Input: dimensioned drawing with shaded views. Units: mm. Origin: part minimum x, y, z. A direction names the side the tool comes from. Give positions to 0.01 mm unless a question says otherwise; leave off trailing zeros. Order: outer loops, then holes, each group sorted by start corner. A loop starts at its lowest first (then second) coordinate and runs counter-clockwise, first axis right, second up.
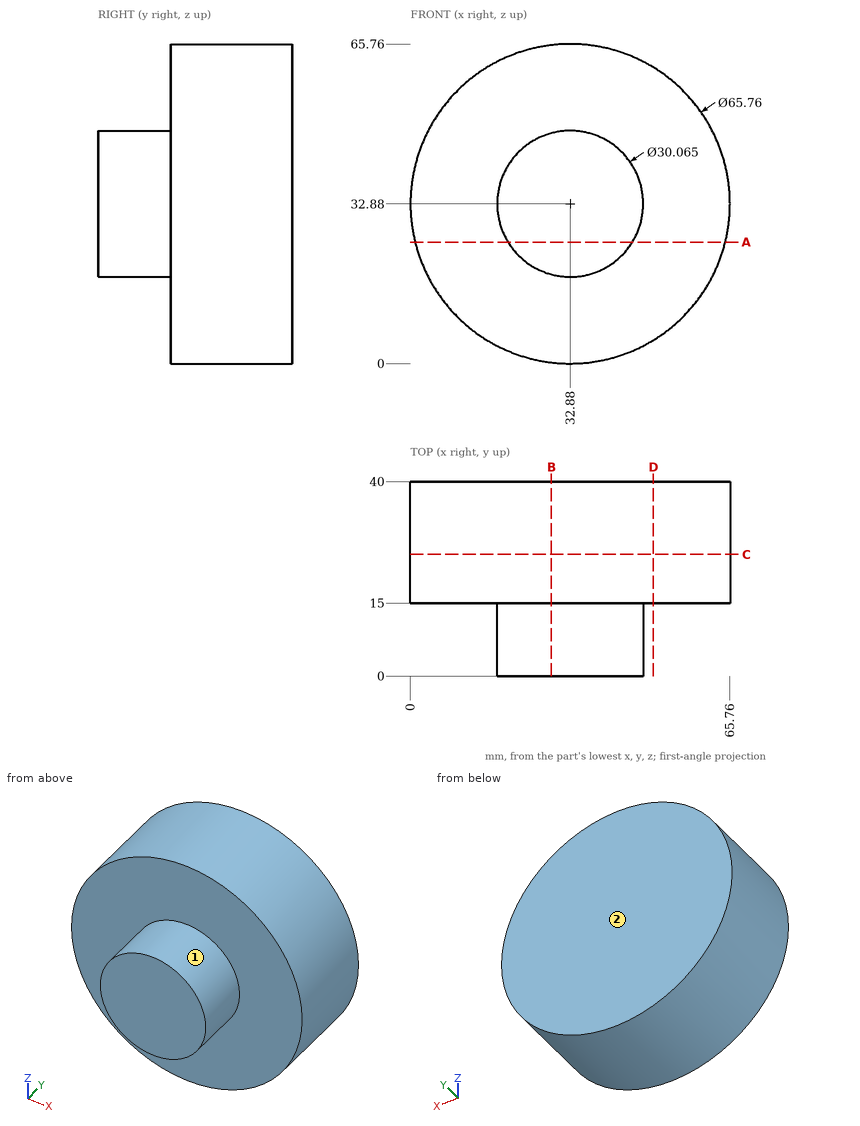
1) Material intervals for L1, parallel to Y at x = 6.5, z = 39.5; L2, parallel to Z at x = 11.5, y = 22; L3, parallel to Z at x = 13.5, y = 37, sorted ascending.
Report:
L1: y = 15 to 40
L2: z = 7.9 to 57.86
L3: z = 6.32 to 59.44
2) Section query A-A, the plane z = 25. Return the cut outline in (x, y), and give its area (3 significant figures).
Report:
outline: (0.96, 15) - (20.08, 15) - (20.08, 0) - (45.68, 0) - (45.68, 15) - (64.8, 15) - (64.8, 40) - (0.96, 40) - close
area: 1,980 mm2
3) Reachability of the marked faces 1 and 2 from +Z, -Z, +X, -X, +Y, -Y: full face, straight path, thin tool, end or side. Return the list, or none.
Report:
face 1: -Y
face 2: +Z, -Z, +X, -X, +Y
4) Pin query (flat end, axial travel): pin 1 (1.5 mm diameter, centred on x = 31, z = 36.5, fed in from -Y); pin 2 (2 mm diameter, centred on y = 29.5, z = 31.5, fed in from -X); pin 3 (6 mm diameter, centred on x = 40, y = 25.5, fed in from +Z); pin 4 (6 mm diameter, centred on y = 7.5, z = 42.5, fed in from +X). Return the tip coordinate at first contact, or that it passes through.
Report:
pin 1: stops at y = 0
pin 2: stops at x = 0
pin 3: stops at z = 65.5
pin 4: stops at x = 46.38
5) Section query C-C, the plane y = 25. Return the cut outline in (x, z).
Report:
outline: circle Ø65.76 at (32.88, 32.88)
6) Section query B-B, the plane x = 29. Return the cut outline in (y, z), and give its area (3 significant figures).
Report:
outline: (0, 18.36) - (15, 18.36) - (15, 0.23) - (40, 0.23) - (40, 65.53) - (15, 65.53) - (15, 47.4) - (0, 47.4) - close
area: 2,070 mm2
7) Section query D-D, the plane x = 50. Return the cut outline in (y, z).
Report:
outline: (15, 4.81) - (40, 4.81) - (40, 60.95) - (15, 60.95) - close
